from build123d import *

# Parameters (mm, degrees)
F1_DEPTH     = 20
F3_DEPTH     = 10
F4_R         = 1.25
F5_DEPTH     = 2.2
F7_DEPTH     = 10
F9_R         = 1.25
F10_DEPTH    = 28.001
F11_R        = 2
F14_DEPTH    = 1.5
F16_W        = 20
F16_H        = 10
F17_DEPTH    = 26.7
F19_R        = 1.25
F20_DEPTH    = 32.1
F22_W        = 20
F22_H        = 9.2705127583
F23_DEPTH    = 6.9
F24_DEPTH    = 2.9
F25_R        = 1.25
F26_DEPTH    = 12.5
F27_W        = 15.1660433039
F27_H        = 51.5122525394
F28_DEPTH    = 40.7
F29_W        = 35.2513279067
F29_H        = 19.1500885412
F30_DEPTH    = 12.5
F31_T1_DEPTH = 17.8
F31_T3_DEPTH = 19.5
F31_T5_DEPTH = 19.3219931649


# Not quite as in the source:
# - a fillet or chamfer that OpenCascade refuses, or shapes differently, is made with other operations: its cross-section is extruded or revolved along the edge and cut away or added


with BuildPart() as f1:
    # F0 (on Top) → F1 (new body)
    with BuildSketch(Plane.XY):
        with BuildLine():
            Line((-17.4218026286, 7.8075558554), (-19.6106751933, 7.8075558554))
            ThreePointArc((-19.6106751933, 7.8075558554), (-13.947676921, -0.1749805422), (-8.2846786486, 7.8075558554))
            Line((-8.2846786486, 7.8075558554), (-10.4735512133, 7.8075558554))
            ThreePointArc((-10.4735512133, 7.8075558554), (-13.947676921, 1.8250194578), (-17.4218026286, 7.8075558554))
        make_face()
    extrude(amount=F1_DEPTH)

    # F2 (on Top) → F3 (join, symmetric)
    with BuildSketch(Plane.XY):
        Polygon((-3.947676921, 1.8250194578), (-13.947676921, 1.8250194578), (-23.947676921, 1.8250194578), (-23.947676921, -1.1749805422), (-3.947676921, -1.1749805422), align=None)
    extrude(amount=F3_DEPTH, both=True)

    # F4 (on Front) → F5 (cut, symmetric)
    with BuildSketch(Plane.XZ):
        with Locations((-11.5779312328, -6)):
            Circle(F4_R)
        with Locations((-21.0779312328, -6)):
            Circle(F4_R)
    extrude(amount=F5_DEPTH, both=True, mode=Mode.SUBTRACT)

    # F6 (on face) → F7 (join, through all)
    with BuildSketch(Plane.XY.offset(10)):
        with BuildLine():
            Line((-3.947676921, 1.8250194578), (-9.475540966, 1.8250194578))
            ThreePointArc((-9.475540966, 1.8250194578), (-13.947676921, -0.1749805422), (-18.419812876, 1.8250194578))
            Line((-18.419812876, 1.8250194578), (-23.947676921, 1.8250194578))
            Line((-23.947676921, 1.8250194578), (-23.947676921, -1.1749805422))
            Line((-23.947676921, -1.1749805422), (-3.947676921, -1.1749805422))
            Line((-3.947676921, -1.1749805422), (-3.947676921, 1.8250194578))
        make_face()
    extrude(amount=F7_DEPTH)

    # F9 (on offset) → F10 (cut, through all)
    with BuildSketch(Plane(origin=(0, 26.8250194578, 0), x_dir=(-1, 0, 0), z_dir=(0, 1, 0))):
        with Locations((23.947676921, -6)):
            Circle(F9_R)
        with Locations((3.947676921, -6)):
            Circle(F9_R)
    extrude(amount=-F10_DEPTH, mode=Mode.SUBTRACT)

    # F11
    f11_edges = [f1.edges().sort_by_distance(p)[0] for p in [
        (-23.947677, 0.325019, -10),
        (-3.947677, 0.325019, -10),
    ]]
    fillet(f11_edges, radius=F11_R)

    # F13 (on offset) → F14 (join)
    with BuildSketch(Plane.XZ.offset(1.1749805422)):
        with BuildLine():
            ThreePointArc((-23.947676921, -4.75), (-22.697676921, -6), (-23.947676921, -7.25))
            Line((-23.947676921, -7.25), (-23.947676921, -8))
            ThreePointArc((-23.947676921, -8), (-23.3618904833, -9.4142135624), (-21.947676921, -10))
            Line((-21.947676921, -10), (-5.947676921, -10))
            ThreePointArc((-5.947676921, -10), (-4.5334633586, -9.4142135624), (-3.947676921, -8))
            Line((-3.947676921, -8), (-3.947676921, -7.25))
            ThreePointArc((-3.947676921, -7.25), (-5.197676921, -6), (-3.947676921, -4.75))
            Line((-3.947676921, -4.75), (-3.947676921, 20))
            Line((-3.947676921, 20), (-23.947676921, 20))
            Line((-23.947676921, 20), (-23.947676921, -4.75))
        make_face()
    extrude(amount=F14_DEPTH)

    # F16 (on offset) → F17 (cut)
    with BuildSketch(Plane(origin=(0, 26.8250194578, 0), x_dir=(-1, 0, 0), z_dir=(0, 1, 0))):
        with Locations((13.947676921, -5)):
            Rectangle(F16_W, F16_H)
    extrude(amount=-F17_DEPTH, mode=Mode.SUBTRACT)

    # F19 (on offset) → F20 (cut)
    with BuildSketch(Plane.XZ.offset(25)):
        with Locations((-11.5779312328, -6)):
            Circle(F19_R)
        with Locations((-21.0779312328, -6)):
            Circle(F19_R)
    extrude(amount=-F20_DEPTH, mode=Mode.SUBTRACT)

    # F22 (on offset) → F23 (cut)
    with BuildSketch(Plane.XY.offset(11.9)):
        with Locations((-13.947676921, 6.460275837)):
            Rectangle(F22_W, F22_H)
    extrude(amount=-F23_DEPTH, mode=Mode.SUBTRACT)

    # F22 (on offset) → F24 (cut)
    with BuildSketch(Plane.XY.offset(11.9)):
        with Locations((-13.947676921, 6.460275837)):
            Rectangle(F22_W, F22_H)
    extrude(amount=F24_DEPTH, mode=Mode.SUBTRACT)

    # F25 (on offset) → F26 (cut, symmetric)
    with BuildSketch(Plane(origin=(0, 1.8250194578, 0), x_dir=(-1, 0, 0), z_dir=(0, 1, 0))):
        with Locations((8.2846786486, 10.0688289385)):
            Circle(F25_R)
        with Locations((19.6106751933, 10.0688289385)):
            Circle(F25_R)
    extrude(amount=F26_DEPTH, both=True, mode=Mode.SUBTRACT)

    # F27 (on offset) → F28 (cut)
    with BuildSketch(Plane(origin=(0, 26.8250194578, 0), x_dir=(-1, 0, 0), z_dir=(0, 1, 0))):
        with Locations((-0.11521345, 4.9743577838)):
            Rectangle(F27_W, F27_H)
    extrude(amount=-F28_DEPTH, mode=Mode.SUBTRACT)

    # F29 (on face) → F30 (cut, symmetric)
    with BuildSketch(Plane(origin=(0, 1.8250194578, 0), x_dir=(-1, 0, 0), z_dir=(0, 1, 0))):
        with Locations((16.3581850356, 23.1292308308)):
            Rectangle(F29_W, F29_H)
    extrude(amount=F30_DEPTH, both=True, mode=Mode.SUBTRACT)

    # F31: fillet of radius 3 on 3 edges, made by hand

    # F31_s2 → F31_t1 (cut)
    with BuildSketch(Plane.XZ.offset(-7.6250194578)):
        with BuildLine():
            ThreePointArc((-7.4678082019, -7), (-8.3464878583, -9.1213203436), (-10.4678082019, -10))
            Line((-10.4678082019, -10), (-7.4678082019, -10))
            Line((-7.4678082019, -10), (-7.4678082019, -7))
        make_face()
    extrude(amount=F31_T1_DEPTH, mode=Mode.SUBTRACT)

    # F31_s4 → F31_t3 (cut)
    with BuildSketch(Plane.XZ.offset(-9.3250194578)):
        with BuildLine():
            ThreePointArc((-20.947676921, 13.5541865602), (-23.0689972645, 12.6755069038), (-23.947676921, 10.5541865602))
            Line((-23.947676921, 10.5541865602), (-23.947676921, 13.5541865602))
            Line((-23.947676921, 13.5541865602), (-20.947676921, 13.5541865602))
        make_face()
    extrude(amount=F31_T3_DEPTH, mode=Mode.SUBTRACT)

    # F31_s6 → F31_t5 (cut)
    with BuildSketch(Plane.XZ.offset(-9.2360160403)):
        with BuildLine():
            ThreePointArc((-10.4322068349, 13.5541865602), (-8.4805938304, 12.8326085319), (-7.4678082019, 11.0149910141))
            Line((-7.4678082019, 11.0149910141), (-7.4678082019, 13.5541865602))
            Line((-7.4678082019, 13.5541865602), (-10.4322068349, 13.5541865602))
        make_face()
    extrude(amount=F31_T5_DEPTH, mode=Mode.SUBTRACT)


solid = f1.part
CAD build for the part. Positions are in the model's coordinates, mm. A direction names the side the tool comes from. Give positions to 0.01 mm unless a question says otherwise; leave off trailing zeros. Write each loop counter-clockwise with the first axis right and the second up, starting at its lowest first coordinate (ties: lowest second). Pieces come first, ordered by that corner, then holes. Notation, with made-up numbers: M 17.5,26 L 28.5,26 A25 ccw 28.5,51 Z; hole C 83.5,64 d4. An arc over 180 degrees is marked long. Put each result on its own line as item: value. Start each with the question number.
(1) Band-saw the part on C-C, the plane y = 4.75. Write the cut outline in (x, z).
(2) Flat gauge pins, fed straight in: pin 1 Ø5 at (x, y) = (-11, 6.5) entering from +Z; pin 2 Ø3 at (y, z) = (5.5, 4) entering from +X; pin 3 Ø4 at (x, z) = (-21.08, -6) entering from +Y (3 decimals). Where does each tip first touch, or does it go through?
(3) Mould opens along Z. For faces 3 (the face through (-8.5, -0.39, 12.85)), 4 (the face through (-23.948, 0, 3)), 5 (the face through (-20.765, -0.393, 9.59)) say: +Z half, -Z half, draft (parallel to the pull), parting line (faces both ways), or undercut.
(4) Band-saw the part on A-A, the plane z = -6. Write the cut outline in (x, y).
(5) Which spindle directions (+Z, -Z, +X, -X, +Y, -Y) get a long thin tool onto all of the face, cutting with end or side? Do faces 1 (the face through (-16, -2.675, 2)), 2 (the face through (-14, 1, 0)). Say none if no direction does.
(6) Probe L1, parallel to X at y = 0.25, z = 9; L2, parallel to Y at x = -20.25, z = 5.5; L3, parallel to Y at x = -9, z = -0.75. List the from-to ranges inside material, lowest first.
(7) Band-saw the part on B-B, the plane x = -18.75. Write the cut outline in (y, z), and give its area (3 significant figures).
(8) Band-saw the part on D-D, the plane y = 1.25. Write the cut outline in (x, z) (3 decimals), and give its area (3 significant figures).
Response values:
1. outline: M -19.85,0 L -17.8,0 L -17.8,5 L -19.85,5 Z; M -10.09,0 L -8.04,0 L -8.04,5 L -10.09,5 Z
2. pin 1: stops at z = 5
2. pin 2: stops at x = -7.95
2. pin 3: stops at y = 0.125
3. face 3: +Z half
3. face 4: draft
3. face 5: undercut
4. outline: M -22.7,-2.67 L -22.33,-2.67 L -22.33,0.13 L -22.7,0.13 Z; M -19.83,-2.67 L -12.83,-2.67 L -12.83,0.13 L -19.83,0.13 Z; M -10.33,-2.67 L -7.47,-2.67 L -7.47,0.13 L -10.33,0.13 Z
5. face 1: +Z, -Z, +X, -X, -Y
5. face 2: -Z, +X, -X, +Y
6. L1: x = -23.95 to -20.26, -18.96 to -8.93, -7.64 to -7.47
6. L2: y = -2.67 to 1.83
6. L3: y = -2.67 to 0.13
7. outline: M -2.67,-10 L 0.13,-10 L 0.13,0 L 1.83,0 L 1.83,9.16 L -2.67,9.16 Z; M -2.67,10.98 L 1.83,10.98 L 1.83,13.55 L -2.67,13.55 Z; M 2.23,0 L 7.81,0 L 7.81,5 L 2.23,5 Z
7. area: 109 mm2
8. outline: M -23.948,0 L -7.468,0 L -7.468,9.123 A1.25 cw long -7.468,11.015 A3 ccw -10.432,13.554 L -20.948,13.554 A3 ccw -23.948,10.554 Z; hole C -19.611,10.069 d2.5
8. area: 210 mm2
